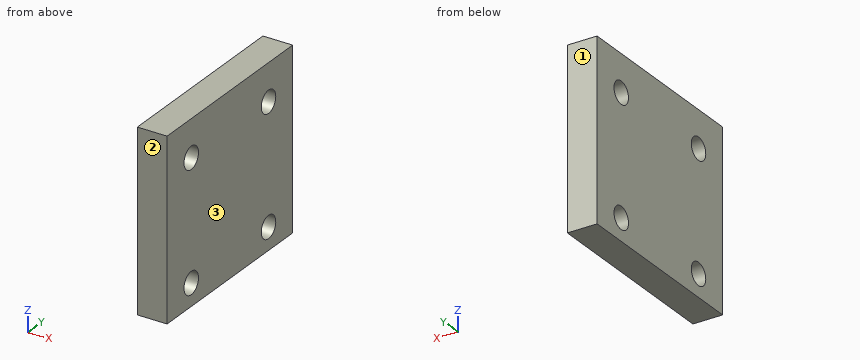
Autodesk Inventor part; units mm, degrees
ref_plane "YZ Plane" through (0, 0, 0) normal (1, 0, 0) x (0, 1, 0)
ref_plane "XZ Plane" through (0, 0, 0) normal (0, 1, 0) x (-1, 0, 0)
ref_plane "XY Plane" through (0, 0, 0) normal (0, 0, 1) x (1, 0, 0)
sketch "Sketch1" plane through (0, 0, 0) normal (1, 0, 0) x (0, 1, 0)
  line L0 (-12.564, -8.5827) -> (20.456, -8.5827)
  line L1 (20.456, -8.5827) -> (20.456, 21.8973)
  line L2 (20.456, 21.8973) -> (-12.564, 21.8973)
  line L3 (-12.564, 21.8973) -> (-12.564, -8.5827)
  point P0 (0, 0)
  dimension "d0" = 30.48
  dimension "d1" = 33.02
extrude "Extrusion1" add sketch "Sketch1" along normal blind 5.08
sketch "Sketch2" plane through (5.08, 0, 0) normal (1, 0, 0) x (0, 0, -1)
  line L0 (8.5827, -12.564) -> (8.5827, 20.456)
  line L1 (-21.8973, -12.564) -> (8.5827, -12.564)
  line L2 (8.5827, 20.456) -> (-21.8973, 20.456)
  line L3 (-21.8973, 20.456) -> (-21.8973, -12.564)
  point P0 (0, 0)
  point P1 (4.7727, 14.106)
  point P2 (-15.5473, 14.106)
  point P3 (-15.5473, -6.214)
  point P4 (4.7727, -6.214)
  dimension "d4" = 3.81
  dimension "d5" = 3.81
  dimension "d6" = 6.35
  dimension "d7" = 6.35
  dimension "d8" = 6.35
  dimension "d9" = 6.35
  dimension "d10" = 6.35
  dimension "d11" = 6.35
hole "Hole1" at (5.08, 14.106, -4.7727) at (5.08, 14.106, 15.5473) at (5.08, -6.214, 15.5473) at (5.08, -6.214, -4.7727) direction (-1, 0, 0) diameter 3.81 depth 10.9728 tip angle 118.188
properties part number "cLIMPpLATE"
Input: part model. Units: mm. Frame: model coordinates. Face numbers are marked on the shaded views. Give positions to 0.01 mm unless a question says otherwise; leave off trailing zeros. Write each loop counter-clockwise with the first axis right and the second up, starting at its lowest first coordinate (ties: lowest second). Pieces come first, ordered by that corner, then holes. Notation, with made-up numbers: M -25,63.5 L 34,63.5 A16 ccw 34,68.5 Z; hole C 19.5,49.5 d7. An arc over 180 degrees is marked long. Write item = value, one per line. Start each with the question number.
1) Draft query along Y for the marked faces 1, 2 and 3. Return one class per face: +Y half, -Y half, draft (parallel to the pull), parting line (faces both ways), or undercut.
2) Material intervals for line 1 along Z through (x, y) = (1.35, -5); line 2 along Y through (x, z) = (1.45, -4); line 3 along Z through (x, y) = (1.7, 15.5), sorted ascending. Write a range as [from, to].
3) Cut plane B-B on y = 14.5. Return the cut outline in (x, z), then the cut area to 3 significant figures.
4) Cut plane A-A on z = 16.5. Return the cut outline in (x, y), then the cut area to 3 significant figures.
5) Cut plane C-C on x = 3.95. Return the cut outline in (y, z) (3 decimals).
6) First-contact query: pin 1 Ø5 at (y, z) = (-6.21, 15.55) entering from +X; pin 2 Ø3.5 at (y, z) = (-6.21, -4.77) entering from -X. Flat tips, straight axial feed; report the tip coordinate or a pass-through.
Solved:
q1.face_1 = +Y half
q1.face_2 = -Y half
q1.face_3 = draft
q2.line_1 = [-8.58, -6.24], [-3.3, 14.08], [17.02, 21.9]
q2.line_2 = [-12.56, -7.96], [-4.47, 12.36], [15.85, 20.46]
q2.line_3 = [-8.58, -6.07], [-3.47, 14.25], [16.85, 21.9]
q3.outline = M 0,-8.58 L 5.08,-8.58 L 5.08,-6.64 L 0,-6.64 Z; M 0,-2.91 L 5.08,-2.91 L 5.08,13.68 L 0,13.68 Z; M 0,17.41 L 5.08,17.41 L 5.08,21.9 L 0,21.9 Z
q3.area = 117 mm2
q4.outline = M 0,-12.56 L 5.08,-12.56 L 5.08,-7.86 L 0,-7.86 Z; M 0,-4.56 L 5.08,-4.56 L 5.08,12.46 L 0,12.46 Z; M 0,15.76 L 5.08,15.76 L 5.08,20.46 L 0,20.46 Z
q4.area = 134 mm2
q5.outline = M -12.564,-8.583 L 20.456,-8.583 L 20.456,21.897 L -12.564,21.897 Z; hole C -6.214,-4.773 d3.81; hole C -6.214,15.547 d3.81; hole C 14.106,-4.773 d3.81; hole C 14.106,15.547 d3.81
q6.pin_1 = 5.08
q6.pin_2 = through
